from build123d import *

# Parameters (mm, degrees)
F0_W      = 94
F0_H      = 45
F1_DEPTH  = 1
F2_W      = 1
F2_H      = 45
F3_DEPTH  = 16
F4_W      = 94
F4_H      = 17
F5_DEPTH  = 1
F6_W      = 1
F6_H      = 6
F7_DEPTH  = 11
F8_R      = 1.25
F8_R_2    = 1.5
F9_DEPTH  = 25
F10_R     = 2
F12_W     = 19.2678107619
F12_H     = 14.8564111814
F12_W_2   = 16.8835728168
F12_H_2   = 15.2771589719
F13_DEPTH = 25
F14_R     = 1.5
F15_DEPTH = 100
F16_SIZE  = 0.5
F17_R     = 1.5
F18_DEPTH = 100
F19_R     = 1.5
F20_DEPTH = 25


with BuildPart() as f1:
    # F0 (on Front) → F1 (new body)
    with BuildSketch(Plane.XZ):
        Rectangle(F0_W, F0_H)
    extrude(amount=F1_DEPTH)

    # F2 (on face) → F3 (join)
    with BuildSketch(Plane(origin=(0, 0, 0), x_dir=(-1, 0, 0), z_dir=(0, 1, 0))):
        with Locations((-46.5, 0)):
            Rectangle(F2_W, F2_H)
        with Locations((46.5, 0)):
            Rectangle(F2_W, F2_H)
    extrude(amount=F3_DEPTH)

    # F4 (on face) → F5 (join)
    with BuildSketch(Plane.XY.offset(22.5)):
        with Locations((0, 7.5)):
            Rectangle(F4_W, F4_H)
    extrude(amount=-F5_DEPTH)

    # F6 (on face) → F7 (join)
    with BuildSketch(Plane.YZ.offset(47)):
        with Locations((15.5, 16)):
            Rectangle(F6_W, F6_H)
        with Locations((15.5, -16)):
            Rectangle(F6_W, F6_H)
    extrude(amount=F7_DEPTH)

    # F8 (on face) → F9 (cut)
    with BuildSketch(Plane.XZ.offset(-15)):
        with Locations((53.5, 16)):
            Circle(F8_R)
        with Locations((53.5, -16)):
            Circle(F8_R_2)
    extrude(amount=-F9_DEPTH, mode=Mode.SUBTRACT)

    # F10
    f10_edges = [f1.edges().sort_by_distance(p)[0] for p in [
        (58, 15.5, -19),
        (58, 15.5, -13),
        (58, 15.5, 19),
        (58, 15.5, 13),
        (47, 15, -16),
        (47, 15, 16),
    ]]
    fillet(f10_edges, radius=F10_R)

    # F11: F1 across plane


with BuildPart() as f1_1:
    add(f1.part)
    add(f1.part.mirror(Plane.YZ))

    # F12 (on face) → F13 (cut)
    with BuildSketch(Plane.XZ.offset(1)):
        with Locations((56.633905381, -15.0717944093)):
            Rectangle(F12_W, F12_H)
        with Locations((-55.4417864084, -14.8614205141)):
            Rectangle(F12_W_2, F12_H_2)
    extrude(amount=-F13_DEPTH, mode=Mode.SUBTRACT)

    # F14 (on face) → F15 (cut)
    with BuildSketch(Plane(origin=(-47, 0, 0), x_dir=(0, -1, 0), z_dir=(-1, 0, 0))):
        with Locations((-9.5, -16)):
            Circle(F14_R)
    extrude(amount=-F15_DEPTH, mode=Mode.SUBTRACT)

    # F16
    f16_edges = [f1_1.edges().sort_by_distance(p)[0] for p in [
        (-46, 11, -16),
        (46, 11, -16),
    ]]
    chamfer(f16_edges, length=F16_SIZE)

    # F17 (on face) → F18 (cut)
    with BuildSketch(Plane(origin=(-47, 0, 0), x_dir=(0, -1, 0), z_dir=(-1, 0, 0))):
        with Locations((-9.5, 8)):
            Circle(F17_R)
    extrude(amount=-F18_DEPTH, mode=Mode.SUBTRACT)

    # F19 (on face) → F20 (cut)
    with BuildSketch(Plane.XZ.offset(1)):
        with Locations((-42.5, 17)):
            Circle(F19_R)
        with Locations((42.5, 17)):
            Circle(F19_R)
        with Locations((-42.5, 5)):
            Circle(F19_R)
        with Locations((42.5, 5)):
            Circle(F19_R)
    extrude(amount=-F20_DEPTH, mode=Mode.SUBTRACT)


solid = f1_1.part
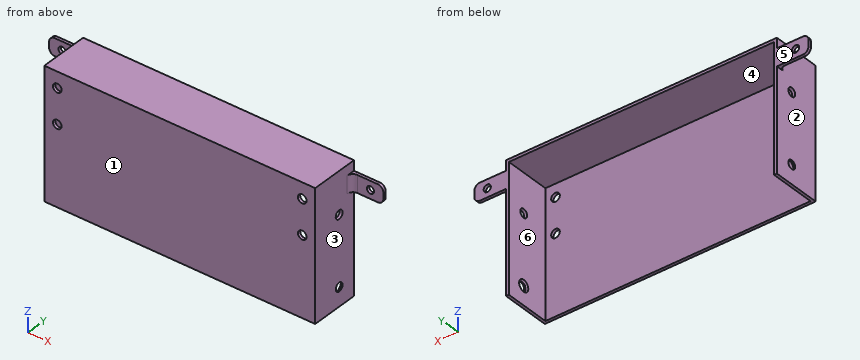
Here's how the part is built. I have some questions about the finished solid (model axes, mm). Face numbers are marked on the shaded views. A direction names the side the tool comes from. Coordinates: 2 decimals unless noted, no trailing zeros. Write each loop counter-clockwise with the first axis right and the second up, starting at its lowest first coordinate (ties: lowest second). Pieces come first, ordered by that corner, then holes.
Item 1: If I drill on line 1 (Z direction, x = 46.8, y = 9.5); line 2 (Z direction, x = 42.5, y = -0.3); line 3 (X direction, y = 8.75, z = 2.5), over which ranges is the centre line in solid material (lowest first)?
Item 2: I want a section at C-C on y = 9.5. Write out the boundary of the cut face in (x, z), and give its area (4 significant figures).
Item 3: On a 3-axis mill with a long thin cutter (end or side, diameter ignored), from which of +Z, -Z, +X, -X, +Y, -Y can I reach the whole of each face in a straight line? I mean the marked faces 5 and 6. Say none if no direction works.
Item 4: If we mould it in two halves opening along X, with no side actions, what happens to the marked faces 1, 2, 3 and 4? For each: +X half, -X half, draft (parallel to the pull), parting line (faces both ways), or undercut.
Item 5: I want a section at D-D on z = -16. Write out the boundary of the cut face in (x, y), and give its area (4 significant figures).
Item 6: I want a section at A-A on z = 5. Write out the boundary of the cut face in (x, y), and give its area (3 significant figures).
Item 7: Will these pins go through, and if not, where does the flat tip stop? pin 1 (5 mm diameter, centred on x = -55.5, z = 16, fed in from -Y); pin 2 (6 mm diameter, centred on y = 5, z = 9.5, fed in from -X); pin 3 (4 mm diameter, centred on y = 11.5, z = 12.5, fed in from +X); pin 4 (10 mm diameter, centred on x = -41, y = 2.5, fed in from -Z).
Item 8: I want a section at B-B on x = 42.5. Write out the boundary of the cut face in (y, z).
Findings below:
1. line 1: z = -22.5 to -17.5, -14.5 to 6.5, 9.5 to 22.5
1. line 2: z = -22.5 to 3.5, 6.5 to 15.5, 18.5 to 22.5
1. line 3: x = -47 to -46, 46 to 47
2. outline: (-47, -22.5) - (-46, -22.5) - (-46, -18) - (-46.5, -17.5) - (-47, -17.5) - close; (-47, -14.5) - (-46.5, -14.5) - (-46, -14) - (-46, 6.5) - (-47, 6.5) - close; (-47, 9.5) - (-46, 9.5) - (-46, 21.5) - (46, 21.5) - (46, 9.5) - (47, 9.5) - (47, 22.5) - (-47, 22.5) - close; (46, -22.5) - (47, -22.5) - (47, -17.5) - (46.5, -17.5) - (46, -18) - close; (46, -14) - (46.5, -14.5) - (47, -14.5) - (47, 6.5) - (46, 6.5) - close
2. area: 169.5 mm2
3. face 5: +Z, -Z, +X, -X, +Y
3. face 6: -Z, +Y
4. face 1: draft
4. face 2: -X half
4. face 3: +X half
4. face 4: undercut
5. outline: (-47, -1) - (47, -1) - (47, 8) - (46.5, 8) - (46, 7.5) - (46, 0) - (-46, 0) - (-46, 7.5) - (-46.5, 8) - (-47, 8) - close; (-47, 11) - (-46.5, 11) - (-46, 11.5) - (-46, 16) - (-47, 16) - close; (46, 11.5) - (46.5, 11) - (47, 11) - (47, 16) - (46, 16) - close
5. area: 119.5 mm2
6. outline: (-47, -1) - (-44, -1) - (-44, 0) - (-46, 0) - (-46, 16) - (-47, 16) - close; (-41, -1) - (41, -1) - (41, 0) - (-41, 0) - close; (44, -1) - (47, -1) - (47, 16) - (46, 16) - (46, 0) - (44, 0) - close
6. area: 120 mm2
7. pin 1: stops at y = 15
7. pin 2: stops at x = -47
7. pin 3: stops at x = 47.05
7. pin 4: stops at z = -22.5
8. outline: (-1, -22.5) - (0, -22.5) - (0, 3.5) - (-1, 3.5) - close; (-1, 6.5) - (0, 6.5) - (0, 15.5) - (-1, 15.5) - close; (-1, 18.5) - (0, 18.5) - (0, 21.5) - (16, 21.5) - (16, 22.5) - (-1, 22.5) - close
